Check sheet for the modelled part. Datum: model origin and axes. Units: mm. Round coordinates to 2 decimals unless told otherwise and drop trailing zeros. Order: outer loops, then holes, each group sorted by start corner. A loop starts at its lowest first (then second) coordinate and runs counter-clockwise, first axis right, second up.
Autodesk Inventor part; units mm, degrees
ref_plane "YZ Plane" through (0, 0, 0) normal (1, 0, 0) x (0, 1, 0)
ref_plane "XZ Plane" through (0, 0, 0) normal (0, 1, 0) x (-1, 0, 0)
ref_plane "XY Plane" through (0, 0, 0) normal (0, 0, 1) x (1, 0, 0)
sketch "Sketch1" plane through (0, 0, 0) normal (0, 1, 0) x (-1, 0, 0)
  circle A0 centre (0, 0) radius 4.25
  dimension "d0" = 8.5
extrude "Extrusion1" add sketch "Sketch1" along normal blind 0.3
sketch "Sketch2" plane through (0, 0.3, 0) normal (0, 1, 0) x (1, 0, 0)
  line L0 (-0.5, 0.5) -> (0.5, 0.5)
  line L1 (0.5, -1.5) -> (0.5, -4.25)
  line L2 (0.5, -4.25) -> (-0.5, -4.25)
  line L3 (-0.5, -4.25) -> (-0.5, -1.5)
  line L4 (-0.5, 0.5) -> (-2.7165, -3.3391)
  line L5 (-2.7165, -3.3391) -> (-1.8505, -3.8391)
  line L6 (-1.8505, -3.8391) -> (-0.5, -1.5)
  line L7 (0.5, -1.5) -> (1.8505, -3.8391)
  line L8 (1.8505, -3.8391) -> (2.7165, -3.3391)
  line L9 (2.7165, -3.3391) -> (0.5, 0.5)
  line L10 (0, 5.95) -> (0, -5.95) construction
  circle A0 centre (0, 0) radius 4.25 construction
  dimension "d3" = 60
  dimension "d4" = 1
  dimension "d5" = 0.5
split_face "Split1"
sketch "Sketch3" plane through (-0.5, 0.3, -0.5) normal (0, 1, 0) x (1, 0, 0)
  line L0 (0, 1) -> (1, 1)
  line L1 (1, 1) -> (1, 3.75)
  line L2 (1, 3.75) -> (0, 3.75)
  line L3 (0, 3.75) -> (0, 1)
  line L4 (0, -4.7205) -> (0, -2)
  line L5 (1, -2) -> (1, -4.7205)
  arc A0 (3.1889, -3.7913) -> (-3.75, -0.5) centre (0.5, -0.5) ccw construction
  line L6 (0, 0) -> (1, 0)
  dimension "d6" = 1
split_face "Split2"
properties part number "Manfrotto Logo 01 - 1"
Item 1: Sectioned sample at A-A (z = 3.75). Record the cut outline in (x, y).
Answer:
outline: (-2, 0) - (2, 0) - (2, 0.3) - (-2, 0.3) - close
Item 2: Sectioned sample at C-C (x = 3). Record the cut outline in (y, z).
Answer:
outline: (0, -3.01) - (0.3, -3.01) - (0.3, 3.01) - (0, 3.01) - close
Item 3: Scan lines: line 1 along Z through (x, y) = (-0.75, 0.15); line 2 along X through (y, z) = (0.2, -2.25). Record each from-to range of solid material in increasing order.
Answer:
line 1: z = -4.18 to 4.18
line 2: x = -3.61 to 3.61
Item 4: Sectioned sample at B-B (y = 0.1). Record the cut outline in (x, z).
Answer:
outline: circle Ø8.5 at (0, 0)
